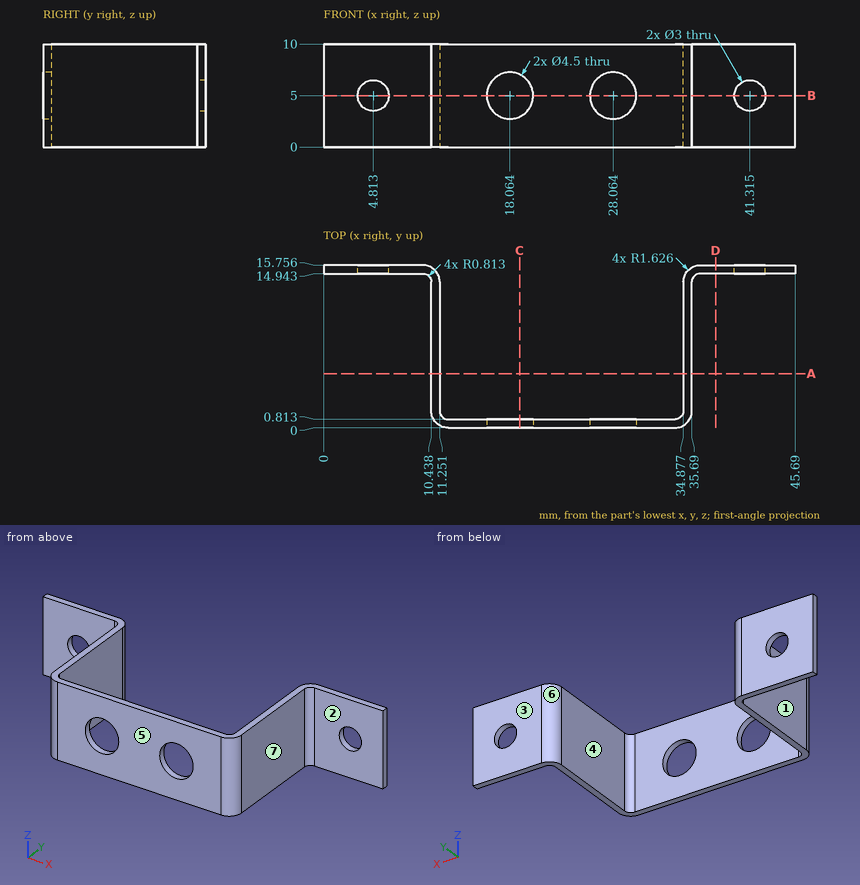
Geometry check sheet. Reference: drawing and pictorial views, mm from the part's lowest x, y, z. A direction names the side the tool comes from. Round coordinates to 2 decimals unless told otherwise and drop trailing zeros. Order: outer loops, then holes, each group sorted by start corner. A loop starts at its lowest first (then second) coordinate and runs counter-clockwise, first axis right, second up. Notation, with made-up numbers: M 65.5,-20 L 81.5,-20 A17 cw 81.5,-2 Z; hole C 70.5,85 d8. An arc over 180 degrees is marked long. One line per item, written item: value. Start each with the question number.
1. Release check for a two-part mould opening along X. For the marked faces 5, 6 and 7 record: released by +X, released by -X, zero draft, split by the parting line, or undercut.
2. Section check D-D on x = 38. Enter the section's corners in (y, z) (1 decimal).
3. Section check B-B on z = 5. Give the number of separate pieces and of enclosed holes in the cut face.
4. Scan lines: line 1 along X through (y, z) = (4.75, 4); line 2 along X through (y, z) = (15.5, 5) (1 decimal); line 3 along X through (y, z) = (0.6, 5) (1 decimal). Record each from-to range of solid material in increasing order.
5. Section check A-A on y = 5.25. Enter the section's corners in (x, z).
6. Gauge pin test, flat ends, axial feed: P1, Ø3, axis at x = 6.5, z = 4.5, coming from the -Y side; P2, Ø3, axis at y = 6.5, z = 6, coming from the +X side; P3, Ø6, axis at x = 18.064, z = 5, coming from the -Y side; P4, Ø4, axis at y = 10, z = 3.5, coming from the -X side. Record the tip position at first contact, or that the pin passes through.
7. Access from +Z, -Z, +X, -X, +Y, -Y to the whole of each face (thin tool, end or side, straight path). Record for the marked faces 1, 2, 3 and 4.
8. Section check C-C on x = 19. Enter the section's corners in (y, z).
Results found:
1. face 5: zero draft
1. face 6: undercut
1. face 7: released by +X
2. outline: M 14.9,0 L 15.8,0 L 15.8,10 L 14.9,10 Z
3. separate pieces: 5
3. enclosed holes: 0
4. line 1: 10.44 to 11.25, 34.88 to 35.69
4. line 2: 0 to 3.3, 6.3 to 10.5, 35.6 to 39.8, 42.8 to 45.7
4. line 3: 10.8 to 15.8, 20.3 to 25.8, 30.3 to 35.3
5. outline: M 10.44,0 L 11.25,0 L 11.25,10 L 10.44,10 Z; M 34.88,0 L 35.69,0 L 35.69,10 L 34.88,10 Z
6. P1: y = 14.94
6. P2: x = 35.69
6. P3: y = 0
6. P4: x = 10.44
7. face 1: +Z, -Z, -X, -Y
7. face 2: +Z, -Z, +X, -Y
7. face 3: +Z, -Z, +X, -X, +Y
7. face 4: +Z, -Z, +Y
8. outline: M 0,0 L 0.81,0 L 0.81,2.95 L 0,2.95 Z; M 0,7.05 L 0.81,7.05 L 0.81,10 L 0,10 Z
